Autodesk Inventor part; units mm, degrees
ref_plane "YZ Plane" through (0, 0, 0) normal (1, 0, 0) x (0, 1, 0)
ref_plane "XZ Plane" through (0, 0, 0) normal (0, 1, 0) x (-1, 0, 0)
ref_plane "XY Plane" through (0, 0, 0) normal (0, 0, 1) x (1, 0, 0)
sketch "Sketch1" plane through (0, 0, 0) normal (0, 0, 1) x (1, 0, 0)
  line L0 (0, 0) -> (0, 14.3)
  line L1 (107.55, 10) -> (107.55, 9.5)
  line L2 (107.55, 9.5) -> (108.65, 9.5)
  line L3 (108.65, 9.5) -> (108.65, 10)
  line L4 (108.65, 10) -> (110.65, 10)
  line L5 (110.65, 0) -> (0, 0)
  line L6 (39.95, 10) -> (39.95, 27.75)
  line L7 (39.95, 27.75) -> (34.95, 27.75)
  line L8 (0, 14.3) -> (2, 14.3)
  line L9 (2, 14.3) -> (2, 13.8)
  line L10 (2, 13.8) -> (3.1, 13.8)
  line L11 (3.1, 13.8) -> (3.1, 14.3)
  line L12 (3.1, 14.3) -> (34.95, 14.3)
  line L13 (34.95, 14.3) -> (34.95, 27.75)
  line L14 (107.55, 10) -> (92.45, 10)
  line L15 (92.45, 10) -> (92.45, 9.5)
  line L16 (92.45, 9.5) -> (91.35, 9.5)
  line L17 (91.35, 9.5) -> (91.35, 10)
  line L18 (110.65, 10) -> (110.65, 0)
  line L19 (91.35, 10) -> (86.025, 10)
  line L20 (86.025, 10) -> (86.025, 9.5)
  line L21 (86.025, 9.5) -> (84.925, 9.5)
  line L22 (84.925, 9.5) -> (84.925, 10)
  line L23 (39.95, 10) -> (44.85, 10)
  line L24 (44.85, 10) -> (44.85, 9.5)
  line L25 (44.85, 9.5) -> (45.95, 9.5)
  line L26 (45.95, 9.5) -> (45.95, 10)
  line L27 (45.95, 10) -> (84.925, 10)
  dimension "d3" = 1.1
  dimension "d6" = 10
  dimension "d8" = 5
  dimension "d9" = 67.6
  dimension "d10" = 27.75
  dimension "d15" = 1.1
  dimension "d16" = 0.5
  dimension "d17" = 2
  dimension "d18" = 31.85
  dimension "d19" = 14.3
  dimension "d20" = 0.5
  dimension "d22" = 0.5
  dimension "d23" = 2
  dimension "d39" = 1.1
  dimension "d40" = 0.5
  dimension "d41" = 15.1
  dimension "d43" = 1.1
  dimension "d44" = 0.5
  dimension "d45" = 44.975
  dimension "d47" = 1.1
  dimension "d48" = 0.5
  dimension "d49" = 6
revolve "Revolution1" add sketch "Sketch1" angle 360 about axis through (110.65, 0, 0) along (-1, 0, 0)
sketch "Sketch2" plane through (39.95, 0, 0) normal (1, 0, 0) x (0, 0, -1)
  arc A0 (19.9153, -3.9332) -> (19.9669, 3.6623) centre (0, 0) ccw
  arc A1 (20.9085, 5.1405) -> (19.9669, 3.6623) centre (21.2333, 3.8946) ccw
  line L0 (20.9085, 5.1405) -> (23.1638, 5.7284)
  arc A2 (24.7533, 4.7239) -> (23.1638, 5.7284) centre (23.4886, 4.4826) ccw
  arc A3 (24.6868, -5.0596) -> (24.7533, 4.7239) centre (0, 0) ccw
  arc A4 (23.0839, -6.0425) -> (24.6868, -5.0596) centre (23.4256, -4.8011) ccw
  line L1 (23.0839, -6.0425) -> (20.8368, -5.424) construction
  arc A5 (19.9153, -3.9332) -> (20.8368, -5.424) centre (21.1784, -4.1826) ccw
  circle A6 centre (20.5409, -12.046) radius 2.1526 construction
  arc A7 (25.2444, 4.8176) -> (23.0377, 6.2122) centre (23.4886, 4.4826) ccw
  line L2 (23.0377, 6.2122) -> (20.7824, 5.6243)
  arc A8 (20.7824, 5.6243) -> (19.4751, 3.5721) centre (21.2333, 3.8946) ccw
  arc A9 (19.4248, -3.8363) -> (19.4751, 3.5721) centre (0, 0) ccw
  arc A10 (19.4248, -3.8363) -> (20.7041, -5.906) centre (21.1784, -4.1826) ccw
  line L3 (20.7041, -5.906) -> (22.9512, -6.5245)
  arc A11 (22.9512, -6.5245) -> (25.1767, -5.16) centre (23.4256, -4.8011) ccw
  arc A12 (25.1767, -5.16) -> (25.2444, 4.8176) centre (0, 0) ccw
  circle A13 centre (20.5409, -12.046) radius 2.6526
  arc A14 (17.126, 16.6141) -> (17.057, 19.2236) centre (15.8707, 17.8866) ccw
  line L4 (15.4668, 14.9772) -> (17.126, 16.6141)
  arc A15 (13.0347, 14.9042) -> (15.4668, 14.9772) centre (14.2115, 16.2497) ccw
  arc A16 (13.0347, 14.9042) -> (6.644, 18.652) centre (0, 0) ccw
  arc A17 (5.5204, 20.8102) -> (6.644, 18.652) centre (7.2438, 20.3359) ccw
  line L5 (6.1389, 23.0574) -> (5.5204, 20.8102)
  arc A18 (8.45, 24.2711) -> (6.1389, 23.0574) centre (7.8623, 22.583) ccw
  arc A19 (17.057, 19.2236) -> (8.45, 24.2711) centre (0, 0) ccw
  circle A20 centre (20.7026, 11.7659) radius 2.6526
  arc A21 (-5.8252, 23.1386) -> (-8.1196, 24.3836) centre (-7.5549, 22.6877) ccw
  line L6 (-5.2373, 20.8833) -> (-5.8252, 23.1386)
  arc A22 (-6.3901, 18.7405) -> (-5.2373, 20.8833) centre (-6.967, 20.4324) ccw
  arc A23 (-6.3901, 18.7405) -> (-12.8311, 15.0799) centre (0, 0) ccw
  arc A24 (-15.262, 15.1859) -> (-12.8311, 15.0799) centre (-13.9895, 16.4412) ccw
  line L7 (-16.8988, 16.8451) -> (-15.262, 15.1859)
  arc A25 (-16.7944, 19.4535) -> (-16.8988, 16.8451) centre (-15.6263, 18.1004) ccw
  arc A26 (-8.1196, 24.3836) -> (-16.7944, 19.4535) centre (0, 0) ccw
  circle A27 centre (0.1617, 23.812) radius 2.6526
  arc A28 (-22.9512, 6.5245) -> (-25.1767, 5.16) centre (-23.4256, 4.8011) ccw
  line L8 (-20.7041, 5.906) -> (-22.9512, 6.5245)
  arc A29 (-19.4248, 3.8363) -> (-20.7041, 5.906) centre (-21.1784, 4.1826) ccw
  arc A30 (-19.4248, 3.8363) -> (-19.4751, -3.5721) centre (0, 0) ccw
  arc A31 (-20.7824, -5.6243) -> (-19.4751, -3.5721) centre (-21.2333, -3.8946) ccw
  line L9 (-23.0377, -6.2122) -> (-20.7824, -5.6243)
  arc A32 (-25.2444, -4.8176) -> (-23.0377, -6.2122) centre (-23.4886, -4.4826) ccw
  arc A33 (-25.1767, 5.16) -> (-25.2444, -4.8176) centre (0, 0) ccw
  circle A34 centre (-20.5409, 12.046) radius 2.6526
  arc A35 (-17.126, -16.6141) -> (-17.057, -19.2236) centre (-15.8707, -17.8866) ccw
  line L10 (-15.4668, -14.9772) -> (-17.126, -16.6141)
  arc A36 (-13.0347, -14.9042) -> (-15.4668, -14.9772) centre (-14.2115, -16.2497) ccw
  arc A37 (-13.0347, -14.9042) -> (-6.644, -18.652) centre (0, 0) ccw
  arc A38 (-5.5204, -20.8102) -> (-6.644, -18.652) centre (-7.2438, -20.3359) ccw
  line L11 (-6.1389, -23.0574) -> (-5.5204, -20.8102)
  arc A39 (-8.45, -24.2711) -> (-6.1389, -23.0574) centre (-7.8623, -22.583) ccw
  arc A40 (-17.057, -19.2236) -> (-8.45, -24.2711) centre (0, 0) ccw
  circle A41 centre (-20.7026, -11.7659) radius 2.6526
  arc A42 (5.8252, -23.1386) -> (8.1196, -24.3836) centre (7.5549, -22.6877) ccw
  line L12 (5.2373, -20.8833) -> (5.8252, -23.1386)
  arc A43 (6.3901, -18.7405) -> (5.2373, -20.8833) centre (6.967, -20.4324) ccw
  arc A44 (6.3901, -18.7405) -> (12.8311, -15.0799) centre (0, 0) ccw
  arc A45 (15.262, -15.1859) -> (12.8311, -15.0799) centre (13.9895, -16.4412) ccw
  line L13 (16.8988, -16.8451) -> (15.262, -15.1859)
  arc A46 (16.7944, -19.4535) -> (16.8988, -16.8451) centre (15.6263, -18.1004) ccw
  arc A47 (8.1196, -24.3836) -> (16.7944, -19.4535) centre (0, 0) ccw
  circle A48 centre (-0.1617, -23.812) radius 2.6526
  point P0 (0, 0)
  dimension "d24" = 0.5
  dimension "d25" = 0.5
  dimension "d28" = 360
extrude "Extrusion1" cut sketch "Sketch2" against normal through all
sketch "Sketch3" plane through (0, 0, 0) normal (-1, 0, 0) x (0, 0, 1)
  circle A0 centre (0, 0) radius 14.3
  point P0 (0, 0)
  point P1 (0, 0)
hole "Hole1" at (0, 0, 0) direction (1, 0, 0) diameter 15 depth 34.95
properties part number "Center Axle" material "Steel, Mild"
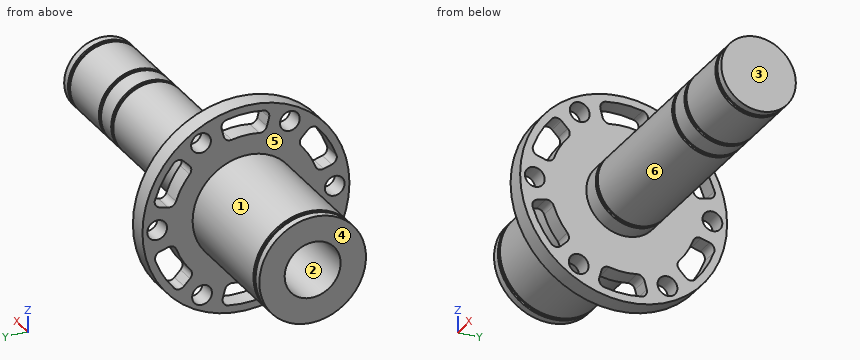
Here's how the part is built. I have some questions about the finished solid (model axes, mm). Face numbers are marked on the shaded views. A direction names the side the tool comes from. Coordinates: 2 decimals unless noted, no trailing zeros. Order: outer loops, then holes, each group sorted by start corner. A loop starts at its lowest first (then second) coordinate and runs counter-clockwise, first axis right, second up.
Item 1: If we mould it in two halves opening along Z, with no side actions, what happens to the marked faces 1, 2 and 3? For each: +Z half, -Z half, draft (parallel to the pull), parting line (faces both ways), or undercut.
Result sheet:
face 1: parting line
face 2: undercut
face 3: draft
Item 2: If we section it at A-A on y = 0: State how many separate pieces and enclosed holes the cut face has, plus the area to 3 significant figures.
Result sheet:
separate pieces: 3
enclosed holes: 0
area: 2,100 mm2
Item 3: If we section it at B-B on x = 11: List the corners of the cut face in (y, z) for me, plus the area to 3 significant figures.
Result sheet:
outline: circle Ø28.6 at (0, 0); hole circle Ø15 at (0, 0)
area: 466 mm2
Item 4: I need wall thicknesses on line 1 (Y direction, x = 36, z = -21.5); line 2 (Y direction, x = 93, z = 7.5); line 3 (X direction, y = -9.5, z = 13). Which ranges of each line are inside material? Lowest first, please.
Result sheet:
line 1: y = -17.54 to -14.52, -9.57 to -6.13, 5.81 to 9.24, 14.3 to 17.54
line 2: y = -6.61 to 6.61
line 3: x = 34.95 to 39.95
Item 5: If we section it at D-D on x = 72.5: List the corners of the cut face in (y, z) for me.
Result sheet:
outline: circle Ø20 at (0, 0)
Item 6: For P1, Ø12, axis at y = -20.5, z = 13.5, coming from the +X side; P2, Ø3, axis at x = 40, y = -12, coming from the +Z side; P3, Ø7, axis at y = 23.81, z = -0.16, coming from the -X side; P4, Ø5, axis at y = 11.77, z = -20.7, coming from the -X side, each with a flat end and sliding along its axis, tell me the tip position at first contact or that it passes through.
Result sheet:
P1: stops at x = 39.95
P2: stops at z = 25.69
P3: stops at x = 34.95
P4: passes through
Item 7: For the marked faces 4, 5 and 6, which set-ups out of +Z, -Z, +X, -X, +Y, -Y let a thin tool reach every point of the face, with its end or its side?
Result sheet:
face 4: +Z, -Z, -X, +Y, -Y
face 5: -X
face 6: +X
